CAD build for the part. Positions are in the model's coordinates, mm. A direction names the side the tool comes from. Round coordinates to 2 decimals unless told otherwise and drop trailing zeros. Order: outer loops, then holes, each group sorted by start corner. A loop starts at its lowest first (then second) coordinate and runs counter-clockwise, first axis right, second up. Notation, with made-up numbers: (61.25, 46.5) -> (90.25, 46.5) arc R17 ccw to (90.25, 78.5) -> close; hole circle Ø4 at (-27, 66). An arc over 180 degrees is marked (long way). Return JSON: item names as keys, results as strings. Group by question number.
Q1. Probe line 1 along Z through (x, y) = (117, 14.5); line 2 along Z through (x, y) = (440, 18.4). List the from-to ranges inside material, lowest first.
Q2. Cut at D-D (x = 206.5). Write the cut outline in (y, z), then the cut area to 3 significant figures.
Q3. Mould opens along Y. For faces 1 (the flat face through (222, 20, 10)), 2 (the flat face through (222, 10, 18)), 3 (the flat face through (450, 1, 10)) say: +Y half, -Y half, draft (parallel to the pull), parting line (faces both ways), or undercut.
Q4. Cut at A-A (z = 10). Write the cut outline in (x, y).
Q5. Cut at C-C (x = 440). Write the cut outline in (y, z).
Q6. Which spindle directions (+Z, -Z, +X, -X, +Y, -Y) get a long thin tool onto all of the face, cutting with end or side? Do faces 4 (the flat face through (222, 18, 10)), 5 (the flat face through (0, 1, 10)). Say none if no direction does.
Q7. Cut at B-B (y = 11.25). Write the cut outline in (x, z).
from build123d import *

# Parameters (mm, degrees)
F0_W     = 20
F0_H     = 20
F0_W_2   = 16
F0_H_2   = 16
F1_DEPTH = 450
F2_R     = 5
F3_DEPTH = 20.001
F4_R     = 5
F5_DEPTH = 20.001


with BuildPart() as f1:
    # F0 (on Right) → F1 (new body)
    with BuildSketch(Plane.YZ):
        with Locations((10, 10)):
            Rectangle(F0_W, F0_H)
        with Locations((10, 10)):
            Rectangle(F0_W_2, F0_H_2, mode=Mode.SUBTRACT)
    extrude(amount=F1_DEPTH)

    # F2 (on face) → F3 (cut, through all)
    with BuildSketch(Plane.XZ):
        with Locations((440, 10)):
            Circle(F2_R)
    extrude(amount=-F3_DEPTH, mode=Mode.SUBTRACT)

    # F4 (on face) → F5 (cut, through all)
    with BuildSketch(Plane.XZ):
        with Locations((10, 10)):
            Circle(F4_R)
    extrude(amount=-F5_DEPTH, mode=Mode.SUBTRACT)


solid = f1.part
Solution:
{
 "1": {"line 1": "z = 0 to 2, 18 to 20", "line 2": "z = 0 to 5, 15 to 20"},
 "2": {"outline": "(0, 0) -> (20, 0) -> (20, 20) -> (0, 20) -> close; hole (2, 2) -> (18, 2) -> (18, 18) -> (2, 18) -> close", "area": "144 mm²"},
 "3": {"face 1": "+Y half", "face 2": "undercut", "face 3": "draft"},
 "4": {"outline": "(0, 0) -> (5, 0) -> (5, 2) -> (0, 2) -> close; (0, 18) -> (5, 18) -> (5, 20) -> (0, 20) -> close; (15, 0) -> (435, 0) -> (435, 2) -> (15, 2) -> close; (15, 18) -> (435, 18) -> (435, 20) -> (15, 20) -> close; (445, 0) -> (450, 0) -> (450, 2) -> (445, 2) -> close; (445, 18) -> (450, 18) -> (450, 20) -> (445, 20) -> close"},
 "5": {"outline": "(0, 0) -> (20, 0) -> (20, 5) -> (18, 5) -> (18, 2) -> (2, 2) -> (2, 5) -> (0, 5) -> close; (0, 15) -> (2, 15) -> (2, 18) -> (18, 18) -> (18, 15) -> (20, 15) -> (20, 20) -> (0, 20) -> close"},
 "6": {"face 4": "+X, -X", "face 5": "+Z, -Z, -X, +Y, -Y"},
 "7": {"outline": "(0, 0) -> (450, 0) -> (450, 2) -> (0, 2) -> close; (0, 18) -> (450, 18) -> (450, 20) -> (0, 20) -> close"}
}
